```python
from build123d import *

# Parameters (mm, degrees)
F1_DEPTH = 10
F3_DEPTH = 3
F4_W     = 35
F4_H     = 20
F5_DEPTH = 25
F6_R     = 4
F7_R     = 4
F8_R     = 4


with BuildPart() as f1:
    # F0 (on Front) → F1 (new body)
    with BuildSketch(Plane.XZ):
        Polygon((64, 0), (0, 0), (0, -2), (0, -39), (15, -49), (32, -49), (49, -49), (64, -39), align=None)
        Polygon((2, -37.5), (2, -2), (62, -2), (62, -37.5), (47.5, -47), (32, -47), (16.5, -47), align=None, mode=Mode.SUBTRACT)
    extrude(amount=F1_DEPTH)

    # F2 (on face) → F3 (join)
    with BuildSketch(Plane.XZ.offset(10)):
        Polygon((0, -39), (15, -49), (49, -49), (64, -39), (64, 0), (0, 0), align=None)
    extrude(amount=F3_DEPTH)

    # F4 (on face) → F5 (cut)
    with BuildSketch(Plane.XZ.offset(13)):
        with Locations((32, -19.5)):
            Rectangle(F4_W, F4_H)
    extrude(amount=-F5_DEPTH, mode=Mode.SUBTRACT)

    # F6
    f6_edges = [f1.edges().sort_by_distance(p)[0] for p in [
        (64, -6.5, 0),
    ]]
    fillet(f6_edges, radius=F6_R)

    # F7
    f7_edges = [f1.edges().sort_by_distance(p)[0] for p in [
        (0, -6.5, 0),
        (64, -6.5, -39),
        (49, -6.5, -49),
        (15, -6.5, -49),
        (0, -6.5, -39),
    ]]
    fillet(f7_edges, radius=F7_R)

    # F8
    f8_edges = [f1.edges().sort_by_distance(p)[0] for p in [
        (2, -5, -2),
        (2, -5, -37.5),
        (62, -5, -2),
        (62, -5, -37.5),
        (47.5, -5, -47),
        (16.5, -5, -47),
    ]]
    fillet(f8_edges, radius=F8_R)


solid = f1.part
```
Check sheet for the modelled part. Datum: model origin and axes. Units: mm. A direction names the side the tool comes from. Give positions to 0.01 mm unless a question says otherwise; leave off trailing zeros. Write each loop counter-clockwise with the first axis right and the second up, starting at its lowest first coordinate (ties: lowest second). Pieces come first, ordered by that corner, then holes.
Item 1: Scan lines: L1, parallel to Z at x = 25, y = -3; L2, parallel to Z at x = 33, y = -10.75; L3, parallel to X at y = -7, z = -18.5. Record each from-to range of solid material in increasing order.
Item 2: Draft check along Z on faces 4 (the face through (32, -5, -2)), 5 (the face through (63.54, -6.59, -38.72)), 6 (the face through (2.49, -5.07, -37.26)), 7 (the face through (64, -6, -21)). Enter one of: released by +Z, released by -Z, zero draft, split by the parting line, or undercut.
Item 3: Access from +Z, -Z, +X, -X, +Y, -Y to the whole of each face (thin tool, end or side, straight path). Record for faces 1 (the face through (62.797, -6.409, -1.141)), 2 (the face through (32, -12, -9.5)), 3 (the face through (60.797, -5.07, -3.141)).
Item 4: Gauge pin test, flat ends, axial feed: pin 1 (3 mm diameter, centred on y = -11, z = -39.5, fed in from +X); pin 2 (10 mm diameter, centred on x = 44.5, z = -12, fed in from +Y); pin 3 (3 mm diameter, centred on x = 9.5, y = -10.5, fed in from -Z). Record the tip position at first contact, or that the pin passes through.
Item 5: Cross-section at D-D (z = -31). Enter the section's corners in (x, y), and give its area (3 significant figures).
Item 6: Cross-section at A-A (x = 36). Enter the section's corners in (y, z).
Item 7: Cross-section at C-C (z = -17.5). Enter the section's corners in (x, y).
Item 8: Cross-section at B-B (y = -1.25). Enter the section's corners in (x, z).
Report:
1. L1: z = -49 to -47, -2 to 0
1. L2: z = -49 to -29.5, -9.5 to 0
1. L3: x = 0 to 2, 62 to 64
2. face 4: undercut
2. face 5: released by -Z
2. face 6: undercut
2. face 7: zero draft
3. face 1: +Z, +X, +Y, -Y
3. face 2: +Y, -Y
3. face 3: +Y
4. pin 1: stops at x = 63.83
4. pin 2: stops at y = -10
4. pin 3: stops at z = -46.33
5. outline: (0, -13) - (64, -13) - (64, 0) - (62, 0) - (62, -10) - (2, -10) - (2, 0) - (0, 0) - close
5. area: 232 mm2
6. outline: (-13, -49) - (0, -49) - (0, -47) - (-10, -47) - (-10, -29.5) - (-13, -29.5) - close; (-13, -9.5) - (-10, -9.5) - (-10, -2) - (0, -2) - (0, 0) - (-13, 0) - close
7. outline: (0, -13) - (14.5, -13) - (14.5, -10) - (2, -10) - (2, 0) - (0, 0) - close; (49.5, -13) - (64, -13) - (64, 0) - (62, 0) - (62, -10) - (49.5, -10) - close
8. outline: (0, -36.86) arc R4 ccw to (1.78, -40.19) - (13.99, -48.33) arc R4 ccw to (16.21, -49) - (47.79, -49) arc R4 ccw to (50.01, -48.33) - (62.22, -40.19) arc R4 ccw to (64, -36.86) - (64, -4) arc R4 ccw to (60, 0) - (4, 0) arc R4 ccw to (0, -4) - close; hole (2, -35.34) arc R4 ccw to (3.81, -38.68) - (15.5, -46.35) arc R4 ccw to (17.69, -47) - (46.31, -47) arc R4 ccw to (48.5, -46.35) - (60.19, -38.68) arc R4 ccw to (62, -35.34) - (62, -6) arc R4 ccw to (58, -2) - (6, -2) arc R4 ccw to (2, -6) - close
